```python
from build123d import *

# Parameters (mm, degrees)
SKETCH2_R               = 2.75
BOSS_EXTRUDE1_DEPTH     = 21.5
SKETCH3_R               = 2.75
BOSS_EXTRUDE2_DEPTH     = 2
SKETCH4_W               = 15
SKETCH4_H               = 15
SKETCH4_R               = 3.7
SKETCH4_R_2             = 2.75
BOSS_EXTRUDE3_DEPTH     = 5
SKETCH5_W               = 15
SKETCH5_H               = 15
SKETCH5_R               = 3.7
BOSS_EXTRUDE4_DEPTH     = 100
CUT_EXTRUDE1_DEPTH      = 138.203316286
CUT_EXTRUDE1_DEPTH_BACK = 138.203316286
SKETCH7_W               = 3.75
SKETCH7_H               = 10
BOSS_EXTRUDE5_DEPTH     = 10
SKETCH8_W               = 3.75
SKETCH8_H               = 10
BOSS_EXTRUDE6_DEPTH     = 10
CUT_EXTRUDE2_DEPTH      = 137.811229437
CUT_EXTRUDE2_DEPTH_BACK = 5
SKETCH9_R               = 1.7
BOSS_EXTRUDE7_START     = 1
BOSS_EXTRUDE7_DEPTH     = 1
FILLET1_R               = 2.5
SKETCH11_R              = 4.75
CUT_EXTRUDE3_DEPTH      = 4


with BuildPart() as part:
    # Sketch2 → Boss-Extrude1 (new body)
    with BuildSketch(Plane.XY):
        with BuildLine():
            ThreePointArc((37.5, -7.5), (41.035533906, -6.035533906), (42.5, -2.5))
            Line((42.5, -2.5), (42.5, 17.5))
            ThreePointArc((42.5, 17.5), (41.035533906, 21.035533906), (37.5, 22.5))
            Line((37.5, 22.5), (18.2530456, 22.5))
            ThreePointArc((18.2530456, 22.5), (20.865716684, 7.5), (18.2530456, -7.5))
            Line((18.2530456, -7.5), (37.5, -7.5))
        make_face()
        with Locations((29.682858342, 0)):
            Circle(SKETCH2_R, mode=Mode.SUBTRACT)
        with Locations((29.682858342, 15)):
            Circle(SKETCH2_R, mode=Mode.SUBTRACT)
    extrude(amount=BOSS_EXTRUDE1_DEPTH)

    # Sketch3 → Boss-Extrude2 (add)
    with BuildSketch(Plane.XY.offset(21.5)):
        with BuildLine():
            Line((18.2530456, -7.5), (37.5, -7.5))
            ThreePointArc((37.5, -7.5), (41.035533906, -6.035533906), (42.5, -2.5))
            Line((42.5, -2.5), (42.5, 17.5))
            ThreePointArc((42.5, 17.5), (41.035533906, 21.035533906), (37.5, 22.5))
            Line((37.5, 22.5), (18.2530456, 22.5))
            ThreePointArc((18.2530456, 22.5), (20.865716684, 7.5), (18.2530456, -7.5))
        make_face()
        with Locations((29.682858342, 0)):
            Circle(SKETCH3_R, mode=Mode.SUBTRACT)
        with Locations((29.682858342, 15)):
            Circle(SKETCH3_R, mode=Mode.SUBTRACT)
    extrude(amount=BOSS_EXTRUDE2_DEPTH)

    # Sketch4 → Boss-Extrude3 (add)
    # profile 1 of 3: a face of its own
    with BuildSketch(Plane.XY.offset(23.5)):
        with BuildLine():
            Line((10.25, 0), (10.25, 15))
            Line((10.25, 15), (18.2530456, 22.5))
            ThreePointArc((18.2530456, 22.5), (20.865716684, 7.5), (18.2530456, -7.5))
            Line((18.2530456, -7.5), (10.25, 0))
        make_face()
    # profile 2 of 3: a face of its own
    with BuildSketch(Plane.XY.offset(23.5)):
        with Locations((2.75, 7.5)):
            Rectangle(SKETCH4_W, SKETCH4_H)
        with Locations((2.75, 7.5)):
            Circle(SKETCH4_R, mode=Mode.SUBTRACT)
    # profile 3 of 3: a face of its own
    with BuildSketch(Plane.XY.offset(23.5)):
        with BuildLine():
            Line((37.5, 22.5), (18.2530456, 22.5))
            ThreePointArc((18.2530456, 22.5), (20.865716684, 7.5), (18.2530456, -7.5))
            Line((18.2530456, -7.5), (37.5, -7.5))
            ThreePointArc((37.5, -7.5), (41.035533906, -6.035533906), (42.5, -2.5))
            Line((42.5, -2.5), (42.5, 17.5))
            ThreePointArc((42.5, 17.5), (41.035533906, 21.035533906), (37.5, 22.5))
        make_face()
        with Locations((29.682858342, 15)):
            Circle(SKETCH4_R_2, mode=Mode.SUBTRACT)
        with Locations((29.682858342, 0)):
            Circle(SKETCH4_R_2, mode=Mode.SUBTRACT)
    extrude(amount=BOSS_EXTRUDE3_DEPTH)

    # Sketch5 → Boss-Extrude4 (add)
    with BuildSketch(Plane.XY.offset(28.5)):
        with Locations((2.75, 7.5)):
            Rectangle(SKETCH5_W, SKETCH5_H)
        with Locations((2.75, 7.5)):
            Circle(SKETCH5_R, mode=Mode.SUBTRACT)
    extrude(amount=BOSS_EXTRUDE4_DEPTH)

    # Sketch6 → Cut-Extrude1 (cut, two sides: drawn at the far end of the back side and taken through both)
    with BuildSketch(Plane.XY.offset(128.5).offset(-CUT_EXTRUDE1_DEPTH_BACK)):
        with BuildLine():
            ThreePointArc((2.75, 3.8), (-0.95, 7.5), (2.75, 11.2))
            Line((2.75, 11.2), (2.75, 15))
            Line((2.75, 15), (-4.75, 15))
            Line((-4.75, 15), (-4.75, 0))
            Line((-4.75, 0), (2.75, 0))
            Line((2.75, 0), (2.75, 3.8))
        make_face()
    extrude(amount=CUT_EXTRUDE1_DEPTH + CUT_EXTRUDE1_DEPTH_BACK, mode=Mode.SUBTRACT)

    # Sketch7 → Boss-Extrude5 (add)
    with BuildSketch(Plane.XZ):
        with Locations((4.625, 123.5)):
            Rectangle(SKETCH7_W, SKETCH7_H)
        with Locations((4.625, 28.5)):
            Rectangle(SKETCH7_W, SKETCH7_H)
    extrude(amount=BOSS_EXTRUDE5_DEPTH)

    # Sketch8 → Boss-Extrude6 (add)
    with BuildSketch(Plane(origin=(0, 15, 0), x_dir=(1, 0, 0), z_dir=(0, 1, 0))):
        with Locations((4.625, -123.5)):
            Rectangle(SKETCH8_W, SKETCH8_H)
        with Locations((4.625, -28.5)):
            Rectangle(SKETCH8_W, SKETCH8_H)
    extrude(amount=BOSS_EXTRUDE6_DEPTH)

    # Sketch9 → Cut-Extrude2 (cut, two sides: drawn at the far end of the back side and taken through both)
    with BuildSketch(Plane.ZY.offset(-2.75).offset(-CUT_EXTRUDE2_DEPTH_BACK)):
        with Locations((123.5, -5)):
            Circle(SKETCH9_R)
        with Locations(Location((123.5, 20, 0), (0, 0, 180))):
            Circle(SKETCH9_R)
        with Locations(Location((28.5, 20, 0), (0, 0, 180))):
            Circle(SKETCH9_R)
        with Locations((28.5, -5)):
            Circle(SKETCH9_R)
    extrude(amount=CUT_EXTRUDE2_DEPTH + CUT_EXTRUDE2_DEPTH_BACK, mode=Mode.SUBTRACT)

    # Sketch10 → Boss-Extrude7 (add)
    with BuildSketch(Plane(origin=(0, 0, 23.5), x_dir=(-1, 0, 0), z_dir=(0, 0, -1)).offset(BOSS_EXTRUDE7_START)):
        with BuildLine():
            Line((-2.75, -10), (-2.75, 3.8))
            ThreePointArc((-2.75, 3.8), (-6.45, 7.5), (-2.75, 11.2))
            Line((-2.75, 11.2), (-2.75, 25))
            Line((-2.75, 25), (-6.5, 25))
            Line((-6.5, 25), (-6.5, 15))
            Line((-6.5, 15), (-10.25, 15))
            Line((-10.25, 15), (-18.2530456, 22.5))
            ThreePointArc((-18.2530456, 22.5), (-20.865716684, 7.5), (-18.2530456, -7.5))
            Line((-18.2530456, -7.5), (-10.25, 0))
            Line((-10.25, 0), (-6.5, 0))
            Line((-6.5, 0), (-6.5, -10))
            Line((-6.5, -10), (-2.75, -10))
        make_face()
    extrude(amount=-BOSS_EXTRUDE7_DEPTH)

    # Fillet1
    fillet1_edges = [part.edges().sort_by_distance(p)[0] for p in [
        (4.625, -10, 22.5),
        (4.625, -10, 33.5),
        (4.625, 25, 22.5),
        (4.625, 25, 33.5),
        (4.625, 25, 118.5),
        (4.625, 25, 128.5),
        (4.625, -10, 118.5),
        (4.625, -10, 128.5),
        (10.25, 0, 78.5),
        (10.25, 15, 78.5),
    ]]
    fillet(fillet1_edges, radius=FILLET1_R)

    # Sketch11 → Cut-Extrude3 (cut)
    with BuildSketch(Plane.XY.offset(28.5)):
        with Locations((29.682858342, 15)):
            Circle(SKETCH11_R)
        with Locations((29.682858342, 0)):
            Circle(SKETCH11_R)
    extrude(amount=-CUT_EXTRUDE3_DEPTH, mode=Mode.SUBTRACT)


solid = part.part
```
Read the model definition and answer for the solid it produces. Units are mm, in the model's axes. A direction names the side the tool comes from. Round coordinates to 2 decimals unless told otherwise and drop trailing zeros. Write each loop counter-clockwise with the first axis right and the second up, starting at its lowest first coordinate (ties: lowest second). Pieces come first, ordered by that corner, then holes. Notation, with made-up numbers: (46, 23.25) -> (50, 23.25) arc R12 cw to (50, 34.25) -> close; hole circle Ø1 at (77, -31.75). An arc over 180 degrees is marked (long way). Answer in a Markdown table with one row per item. Add a question column.
1) Find section A-A, the plane x = 5. Determine the outline of the cut face in (y, z).
2) Determine the mould class of faces 1 (the face through (34.214, 16.427, 26.528)), 2 (the face through (5, 24, 128)), 3 (the face through (6.5, -3.8, 26.7)) for opening direction Y: pulls with the +Y half, pulls with the -Y half, needs draft (parallel to the pull), parting line crosses it, or undercut.
3) Given P1, Ø3, axis at y = 20.5, z = 125.5, coming from the +X side; P2, Ø2, axis at x = 5.5, z = 55.5, coming from the -Y side; P3, Ø4.5, axis at x = 29.68, y = 15, coming from the -Z side; P4, Ø21, axis at x = 27, z = 10, coming from the -Y side, each flat-ended and moving along its own axis, determine where each tip first touches the part or whether it passes through.
4) Find section C-C, the plane y = 7.5. Determine the outline of the cut face in (x, z).
5) Consider line 1 (Z direction, x = 5.45, y = -5); line 2 (Y direction, x = 4.45, z = 123.5); line 3 (Y direction, x = 5, z = 123). Determine where each line is inside the solid, lowest interval first.
6) Find section B-B, the plane z = 14.5. Determine the outline of the cut face in (x, y).
7) Find section D-D, the plane z = 123.5. Determine the outline of the cut face in (x, y), and give its area (3 significant figures).
8) Which of the six approach directions +Z, -Z, +X, -X, +Y, -Y give full straight-line access (tool end or side, diameter ignored) to faces 4 (the face through (9.537, 0.752, 79.2)), 5 (the face through (14.308, -3.803, 25.458)), 6 (the face through (5, 19, 33.5)), 7 (the face through (6.5, 19, 26.7))?
Findings below:
| question | item | result |
|---|---|---|
| 1 | outline | (-10, 25) arc R2.5 ccw to (-7.5, 22.5) -> (4.56, 22.5) -> (4.56, 128.5) -> (-7.5, 128.5) arc R2.5 ccw to (-10, 126) -> (-10, 121) arc R2.5 ccw to (-7.5, 118.5) -> (0, 118.5) -> (0, 33.5) -> (-7.5, 33.5) arc R2.5 ccw to (-10, 31) -> close; (10.44, 22.5) -> (22.5, 22.5) arc R2.5 ccw to (25, 25) -> (25, 31) arc R2.5 ccw to (22.5, 33.5) -> (15, 33.5) -> (15, 118.5) -> (22.5, 118.5) arc R2.5 ccw to (25, 121) -> (25, 126) arc R2.5 ccw to (22.5, 128.5) -> (10.44, 128.5) -> close; hole circle Ø3.4 at (-5, 28.5); hole circle Ø3.4 at (-5, 123.5); hole circle Ø3.4 at (20, 28.5); hole circle Ø3.4 at (20, 123.5) |
| 2 | face 1 | undercut |
| 2 | face 2 | pulls with the +Y half |
| 2 | face 3 | needs draft |
| 3 | P1 | x = 6.5 |
| 3 | P2 | y = 0 |
| 3 | P3 | through |
| 3 | P4 | y = -7.5 |
| 4 | outline | (6.45, 22.5) -> (20.87, 22.5) -> (20.87, 0) -> (42.5, 0) -> (42.5, 28.5) -> (10.25, 28.5) -> (10.25, 128.5) -> (6.45, 128.5) -> close |
| 5 | line 1 | 22.5 to 26.8, 30.2 to 33.5, 118.5 to 121.8, 125.2 to 128.5 |
| 5 | line 2 | -10 to -6.7, -3.3 to 4.21, 10.79 to 18.3, 21.7 to 25 |
| 5 | line 3 | -10 to -6.62, -3.38 to 4.56, 10.44 to 18.38, 21.62 to 25 |
| 6 | outline | (18.25, -7.5) -> (37.5, -7.5) arc R5 ccw to (42.5, -2.5) -> (42.5, 17.5) arc R5 ccw to (37.5, 22.5) -> (18.25, 22.5) arc R44.37 cw to start; hole circle Ø5.5 at (29.68, 0); hole circle Ø5.5 at (29.68, 15) |
| 7 | outline | (2.75, -10) -> (6.5, -10) -> (6.5, -6.7) -> (2.75, -6.7) -> close; (2.75, -3.3) -> (6.5, -3.3) -> (6.5, 0) -> (7.75, 0) arc R2.5 ccw to (10.25, 2.5) -> (10.25, 12.5) arc R2.5 ccw to (7.75, 15) -> (6.5, 15) -> (6.5, 18.3) -> (2.75, 18.3) -> (2.75, 11.2) arc R3.7 cw to (2.75, 3.8) -> close; (2.75, 21.7) -> (6.5, 21.7) -> (6.5, 25) -> (2.75, 25) -> close |
| 7 | area | 138 mm² |
| 8 | face 4 | +Z, +X, -Y |
| 8 | face 5 | +Z, -Z, -Y |
| 8 | face 6 | +X, -X, +Y |
| 8 | face 7 | +Z, -Z, +Y |
